Autodesk Inventor part; units mm, degrees
ref_plane "YZ Plane" through (0, 0, 0) normal (1, 0, 0) x (0, 1, 0)
ref_plane "XZ Plane" through (0, 0, 0) normal (0, 1, 0) x (-1, 0, 0)
ref_plane "XY Plane" through (0, 0, 0) normal (0, 0, 1) x (1, 0, 0)
sketch "Sketch1" plane through (0, 0, 0) normal (0, 0, 1) x (1, 0, 0)
  line L0 (1.6454, 2.85) -> (3.2909, 0)
  line L1 (3.2909, 0) -> (1.6454, -2.85)
  line L2 (1.6454, -2.85) -> (-1.6454, -2.85)
  line L3 (-1.6454, -2.85) -> (-1.6498, -2.8425)
  line L4 (-1.6454, 2.85) -> (1.6454, 2.85)
  line L5 (-1.6454, 2.85) -> (-2.5099, 4.3244)
  line L6 (-1.6498, -2.8425) -> (-2.5099, -4.3244)
  line L7 (3.2909, 0) -> (53.2909, 0) construction
  line L8 (5, 0) -> (53.2909, 0) construction
  line L9 (5.3327, -3.25) -> (53.2909, -3.25)
  line L10 (53.2909, 3.25) -> (5.3327, 3.25)
  arc A0 (53.2909, -3.25) -> (53.2909, 3.25) centre (53.2909, 0) ccw
  arc A1 (-2.5099, -4.3244) -> (2.9626, -4.0278) centre (0, 0) ccw
  arc A2 (2.9626, 4.0278) -> (-2.5099, 4.3244) centre (0, 0) ccw
  arc A3 (2.9626, 4.0278) -> (5.3327, 3.25) centre (5.3327, 7.25) ccw
  arc A4 (5.3327, -3.25) -> (2.9626, -4.0278) centre (5.3327, -7.25) ccw
  circle A5 centre (53.2909, 0) radius 1.5
  point P0 (3.7997, 3.25)
  point P1 (29.1454, 0)
  point P2 (3.7997, -3.25)
  dimension "d0" = 5.7
  dimension "d2" = 50
  dimension "d3" = 6.5
  dimension "d4" = 4
  dimension "d5" = 3
extrude "Extrusion1" add sketch "Sketch1" along normal blind 2.4
properties part number "1pcs-m4-wrench"
The listing builds one solid part. Answer for the finished solid, in the listing's coordinates (mm). A direction names the side the tool comes from. Coordinates: 2 decimals unless noted, no trailing zeros. Write each loop counter-clockwise with the first axis right and the second up, starting at its lowest first coordinate (ties: lowest second). Pieces come first, ordered by that corner, then holes. Notation, with made-up numbers: M 58,57.5 L 93,57.5 A28 ccw 93,76.5 Z; hole C 69.5,84.25 d10. An arc over 180 degrees is marked long. Use a Markdown table: item, result. Add a question column.
1. Which of the six approach directions +Z, -Z, +X, -X, +Y, -Y give full straight-line access (tool end or side, diameter ignored) to faces 1 (the flat face through (0, 2.85, 1)), 2 (the flat face through (30, 3.25, 1)), 3 (the flat face through (29, -3.25, 1)), 4 (the cylindrical face through (0, 5, 1)), 5 (the cylindrical face through (56.54, 0.07, 1.18))?
2. For a pull along Y with two mould halves and no side action, classify faces 6 (the flat face through (2.46, 1.44, 1.18)), 7 (the cylindrical face through (0, -5, 1)), 8 (the flat face through (27, 0, 0)), 9 (the flat face through (2.48, -1.405, 1.183)) as +Y half, -Y half, draft (parallel to the pull), parting line (faces both ways), or undercut.
3. Section B-B (x = 18) is taken. Give the vertices of the cut face in (y, z), plus the area to 3 significant figures.
4. Straight lines are drawn through the part: line 1 along Y through (x, z) = (15.5, 1.4); line 2 along X through (y, z) = (-1.25, 0.65); line 3 along Y through (x, z) = (1.5, 1.8). For each, find the intervals that lie inside material, in ascending order. Write a range as [from, to].
5. Given P1, Ø0.7, axis at x = 30.5, z = 1, coming from the -Y side; P2, Ø1, axis at y = -2.5, z = 1, coming from the +X side, each flat-ended and moving along its own axis, determine where each tip first touches the part or whether it passes through.
6. Section C-C (y = 2) is taken. Give the vertices of the cut face in (x, z).
Data:
| question | item | result |
|---|---|---|
| 1 | face 1 | +Z, -Z, -X |
| 1 | face 2 | +Z, -Z, +X, +Y |
| 1 | face 3 | +Z, -Z, +X, -Y |
| 1 | face 4 | +Z, -Z, +Y |
| 1 | face 5 | +Z, -Z, +X |
| 2 | face 6 | undercut |
| 2 | face 7 | -Y half |
| 2 | face 8 | draft |
| 2 | face 9 | undercut |
| 3 | outline | M -3.25,0 L 3.25,0 L 3.25,2.4 L -3.25,2.4 Z |
| 3 | area | 15.6 mm2 |
| 4 | line 1 | y = [-3.25, 3.25] |
| 4 | line 2 | x = [2.57, 52.46], [54.12, 56.29] |
| 4 | line 3 | y = [-4.77, -2.85], [2.85, 4.77] |
| 5 | P1 | stops at y = -3.25 |
| 5 | P2 | stops at x = 55.85 |
| 6 | outline | M 2.14,0 L 55.85,0 L 55.85,2.4 L 2.14,2.4 Z |
